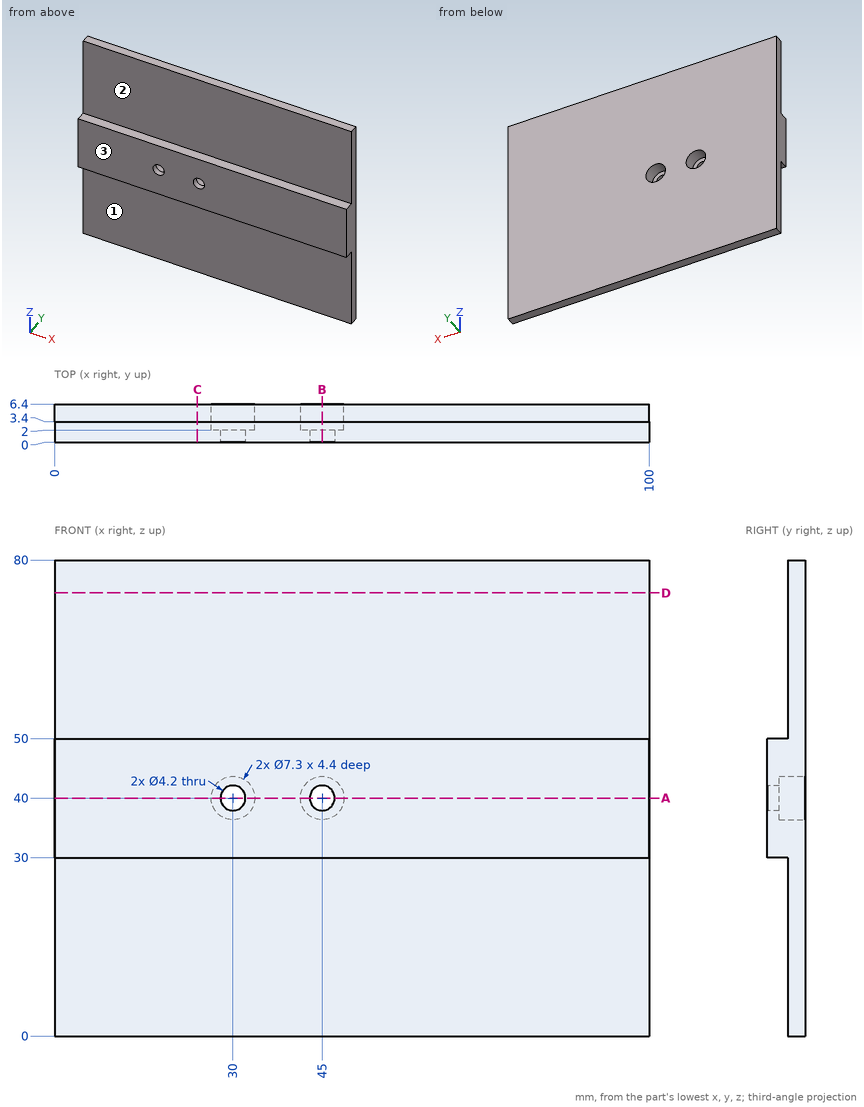
Geometry check sheet. Reference: drawing and pictorial views, mm from the part's lowest x, y, z. A direction names the side the tool comes from. Coordinates: 2 decimals unless noted, no trailing zeros. Write each loop counter-clockwise with the first axis right and the second up, starting at its lowest first coordinate (ties: lowest second). Pieces come first, ordered by that corner, then holes. Notation, with made-up numbers: M 8,55 L 67,55 A20 cw 67,59 Z; hole C 7,82.25 d5. An arc over 180 degrees is marked long. Write item = value, one per line. Start each with the question number.
1. Thickness scan on probe 1 along Z at (x, y) = (30, 5.45); probe 2 along Z at (x, y) = (45, 1.2); probe 3 along Y at (x, z) = (20, 21.5). Record the ranges inside material, lowest first.
2. Tool access check on the marked faces 1, 2 and 3. Record the directions out of +Z, -Z, +X, -X, +Y, -Y that give a thin tool (end or side, any length) a straight path to the whole face; none if there is none.
3. Sectioned sample at B-B (x = 45). Record the cut outline in (y, z).
4. Sectioned sample at A-A (z = 40). Record the cut outline in (x, y).
5. Sectioned sample at D-D (z = 74.5). Record the cut outline in (x, y).
6. Go/stop test with flat-tipped pins: pin 1 (1 mm diameter, centred on x = 36.5, y = 2, fed in from +Z); pin 2 (1 mm diameter, centred on x = 40, y = 2, fed in from -Z); pin 3 (4.5 mm diameter, centred on x = 30, z = 40, fed in from +Y). Record where each tip stops, or that it passes through.
7. Sectioned sample at C-C (x = 24). Record the cut outline in (y, z), then the cut area to 3 significant figures.
The answers:
q1.probe_1 = 0 to 36.35, 43.65 to 80
q1.probe_2 = 30 to 37.9, 42.1 to 50
q1.probe_3 = 3.4 to 6.4
q2.face_1 = -Z, +X, -X, -Y
q2.face_2 = +Z, +X, -X, -Y
q2.face_3 = +Z, -Z, +X, -X, -Y
q3.outline = M 0,30 L 3.4,30 L 3.4,0 L 6.4,0 L 6.4,36.35 L 2,36.35 L 2,37.9 L 0,37.9 Z; M 0,42.1 L 2,42.1 L 2,43.65 L 6.4,43.65 L 6.4,80 L 3.4,80 L 3.4,50 L 0,50 Z
q4.outline = M 0,0 L 27.9,0 L 27.9,2 L 26.35,2 L 26.35,6.4 L 0,6.4 Z; M 32.1,0 L 42.9,0 L 42.9,2 L 41.35,2 L 41.35,6.4 L 33.65,6.4 L 33.65,2 L 32.1,2 Z; M 47.1,0 L 100,0 L 100,6.4 L 48.65,6.4 L 48.65,2 L 47.1,2 Z
q5.outline = M 0,3.4 L 100,3.4 L 100,6.4 L 0,6.4 Z
q6.pin_1 = 50
q6.pin_2 = 30
q6.pin_3 = 2
q7.outline = M 0,30 L 3.4,30 L 3.4,0 L 6.4,0 L 6.4,80 L 3.4,80 L 3.4,50 L 0,50 Z
q7.area = 308 mm²
